Autodesk Fusion 360 part; units mm, degrees
sketch "Sketch2" plane through (0, 0, 0) normal (1, 0, 0) x (0, 1, 0)
  line L0 (0, 0) -> (-113.2, 0)
  line L1 (-113.2, 0) -> (-113.2, 26.7)
  line L2 (-86.3, 51.9) -> (0, 51.9)
  line L3 (0, 51.9) -> (0, 0)
  line L4 (-86.3, 51.9) -> (-113.2, 26.7)
  dimension "d1" = 113.2
  dimension "d2" = 51.9
  dimension "d3" = 86.3
  dimension "d4" = 26.7
extrude "Extrude1" add sketch "Sketch2" along normal blind 62.2 makes body 1
ref_plane "WorkPlane1" through (31.1, 0, 0) normal (1, 0, 0) x (0, 1, 0)
sketch "Sketch3" plane through (31.1, 0, 0) normal (1, 0, 0) x (0, 1, 0)
  line L0 (47.8879, 197.95) -> (-89.5121, 197.95)
  line L1 (-89.5121, 197.95) -> (-89.5121, 163.6)
  line L2 (-89.5121, 163.6) -> (47.8879, 163.6)
  line L3 (47.8879, 163.6) -> (47.8879, 197.95)
  line L4 (0, 51.9) -> (0, 0)
  line L5 (-86.3, 51.9) -> (0, 51.9)
  line L6 (-89.5121, 191) -> (-158.2121, 191)
  line L7 (-158.2121, 191) -> (-158.2121, 163.6)
  line L8 (-158.2121, 163.6) -> (-89.5121, 163.6)
  line L9 (-89.5121, 163.6) -> (-89.5121, 191)
  line L10 (-89.5121, 177.3) -> (-158.2121, 177.3) construction
  line L11 (-158.2121, 191) -> (-213.1721, 191)
  line L12 (-213.1721, 191) -> (-213.1721, 170.45)
  line L13 (-213.1721, 170.45) -> (-158.2121, 170.45)
  line L14 (-158.2121, 170.45) -> (-158.2121, 191)
  line L15 (-213.1721, 170.45) -> (-213.1721, 191)
  line L16 (-213.1721, 191) -> (-229.6121, 191)
  line L17 (-229.6121, 191) -> (-229.6121, 178.3)
  line L18 (-229.6121, 178.3) -> (-213.1721, 170.45)
  spline S0 degree 5 poles (-26.0256, 51.9) (-25.8292, 53.4797) (-25.5289, 56.5687) (-25.3557, 60.9909) (-25.6831, 66.462) (-27.0217, 72.5971) (-29.2397, 78.079) (-32.2063, 83.0319) (-35.6533, 87.7033) (-39.2005, 92.4405) (-42.4377, 97.6159) (-44.9819, 103.5758) (-46.5608, 110.5628) (-47.0265, 118.7038) (-46.3099, 128.0539) (-44.3968, 138.6184) (-41.9207, 148.0265) (-39.5419, 155.6097) (-37.7257, 160.8978) (-36.7601, 163.6) knots 0 0 0 0 0 0 0.066667 0.133333 0.2 0.266667 0.333333 0.4 0.466667 0.533333 0.6 0.666667 0.733333 0.8 0.866667 0.933333 1 1 1 1 1 1 construction
  line L19 (21.6823, 163.6) -> (-88.6177, 163.6)
  line L20 (-88.6177, 163.6) -> (-88.6177, 151.3)
  line L21 (-88.6177, 151.3) -> (21.6823, 151.3)
  line L22 (21.6823, 151.3) -> (21.6823, 163.6)
  line L23 (-14.1079, 151.3) -> (-81.2298, 151.3)
  line L24 (-81.2298, 151.3) -> (-81.2298, 125.6)
  line L25 (-81.2298, 125.6) -> (-14.1079, 125.6)
  line L26 (-14.1079, 125.6) -> (-14.1079, 151.3)
  point P0 (-30.5104, 80)
  point P1 (-43.5557, 100.5876)
  dimension "d8" = 111.7
  dimension "d9" = 34.35
  dimension "d10" = 137.4
  dimension "d11" = 68.7
  dimension "d12" = 27.4
  dimension "d13" = 20.55
  dimension "d14" = 54.96
  dimension "d15" = 20.55
  dimension "d16" = 12.7
  dimension "d17" = 16.44
  dimension "d18" = 110.3
  dimension "d19" = 12.3
  dimension "d20" = 25.7
revolve "Revolve1" add sketch "Sketch3" angle 360 about axis through (31.1, -89.5121, 191) along (0, -1, 0) separate body contours L1 L6 L7 L8 L9 L14 | L7 L11 L12 L13 L14 L15 | L12 L15 L16 L17 L18 makes body 2
revolve "Revolve2" add sketch "Sketch3" angle 360 about axis through (31.1, 47.8879, 197.95) along (0, -1, 0) contours L0 L1 L2 L3 L9 L19 bodies 2
extrude "Extrude2" add sketch "Sketch3" along normal mid plane 23.4 separate body contours L2 L19 L20 L21 L22 L23 makes body 3
extrude "Extrude3" add sketch "Sketch3" along normal mid plane 15.9 contours L21 L23 L24 L25 L26 bodies 3
sketch "Sketch5" plane through (0, 0, 51.9) normal (0, 0, 1) x (-1, 0, 0)
  line L0 (0, 0) -> (0, 86.3)
  line L1 (0, 86.3) -> (-62.2, 86.3)
  line L2 (-62.2, 86.3) -> (-62.2, 0)
  line L3 (-62.2, 0) -> (0, 0)
  ellipse E0 centre (-30, 30) end of major axis (-48.66, 30) minor radius 19.45
  line L4 (-11.34, 30) -> (-48.66, 30) construction
  line L5 (-30, 49.45) -> (-30, 10.55) construction
  dimension "d27" = 38.9
  dimension "d28" = 37.32
sweep "Sweep1" add profiles "Sketch5" path "Sketch3" along S0 section 1 contours E0 bodies 1 2 3
equation "d9 = ( 68.7 / 2 ) * 1 mm"
equation "d10 = ( 2 * 68.7 ) * 1 mm"
equation "d12 = ( 54.8 / 2 ) * 1 mm"
equation "d13 = ( 41.1 / 2 ) * 1 mm"
equation "d14 = ( ( 4 / 5 ) * 68.7 ) * 1 mm"
equation "d15 = ( 41.1 / 2 ) * 1 mm"
equation "d16 = ( 25.4 / 2 ) * 1 mm"
equation "d17 = ( 41.1 * ( 2 / 5 ) ) * 1 mm"
equation "d23 = ( 23.4 / 2 ) * 1 mm"
equation "d25 = ( 15.9 / 2 ) * 1 mm"
equation "d28 = ( ( 3 / 5 ) * 62.2 ) * 1 mm"
Read the model definition and answer for the solid it produces. Units are mm, in the model's axes. A direction names the side the tool comes from. Round coordinates to 2 decimals unless told otherwise and drop trailing zeros. Loops run counter-clockwise (first coordinate to the right, second up) from the corner with the lowest first, then second, coordinate; pieces in that order, holes last.
Q1. Which of the six approach directions +Z, -Z, +X, -X, +Y, -Y give full straight-line access (tool end or side, diameter ignored) to faces 4 (the face through (13.772, -185.307, 179.952)), 5 (the face through (31, -14.108, 138)), 6 (the face through (23.15, -21, 139)), 7 (the face through (39.05, -22, 139)), 8 (the face through (31, -88.618, 158))?
Q2. Determine the mould class of faces 1 (the face through (31, -74, 125.6)), 2 (the face through (30.52, -228.58, 204.18)), 3 (the face through (52, -158.212, 187)) for opening direction Z: released by +Z, released by -Z, zero draft, split by the parting line, or undercut.
Q3. Section C-C on y = -183 is taken. Write down the section's boundary in (x, z), and give its area (3 significant figures).
Q4. Each of these flat-tipped pins is pushed along its axis until it touches: pin 1 (3.5 mm diameter, centred on x = 31.5, z = 155.5, fed in from +Y); pin 2 (5 mm diameter, centred on y = -48, z = 49.5, fed in from +X); pin 3 (5 mm diameter, centred on y = -88.5, z = 36.5, fed in from -X); pin 4 (15.5 mm diameter, centred on x = 30.5, y = -77.5, fed in from -Z). Where does it stop, or does it pass through?
Q5. Consider probe 1 along Y at (x, z) = (52, 197); probe 2 along Z at (x, y) = (32, -198.5); probe 3 along Z at (x, y) = (26.5, -79.5). Determine where each line is inside the solid, lowest interval first.
Q6. Section B-B on z = 191 is taken. Write down the section's boundary in (x, y), and give its area (3 significant figures).
Output:
1. face 4: -Y
1. face 5: +X, -X, +Y
1. face 6: -X, +Y
1. face 7: +X, +Y
1. face 8: +X, -X, -Y
2. face 1: undercut
2. face 2: split by the parting line
2. face 3: zero draft
3. outline: circle Ø41.1 at (31.1, 191)
3. area: 1,330 mm2
4. pin 1: stops at y = 21.68
4. pin 2: stops at x = 62.2
4. pin 3: stops at x = 0
4. pin 4: stops at z = 0
5. probe 1: y = -158.21 to 47.89
5. probe 2: z = 170.47 to 211.53
5. probe 3: z = 0 to 51.9, 125.6 to 163.6, 163.91 to 231.99
6. outline: (-2.54, -89.51) - (3.7, -89.51) - (3.7, -158.21) - (10.55, -158.21) - (10.55, -213.17) - (18.4, -229.61) - (43.8, -229.61) - (51.65, -213.17) - (51.65, -158.21) - (58.5, -158.21) - (58.5, -89.51) - (64.74, -89.51) - (64.74, 47.89) - (-2.54, 47.89) - close
6. area: 15,800 mm2
